```python
from build123d import *

# Parameters (mm, degrees)
SKETCH1_R                                    = 17.5
SKETCH1_R_2                                  = 8
BOSS_EXTRUDE1_DEPTH                          = 2
CSK_FOR_M3_COUNTERSUNK_FLAT_HEAD_SCR_2_COUNT = 2
CSK_FOR_M3_COUNTERSUNK_FLAT_HEAD_SCR_2_PITCH = 19.902355243
CSK_FOR_M3_COUNTERSUNK_FLAT_HEAD_SCR_3_COUNT = 2
CSK_FOR_M3_COUNTERSUNK_FLAT_HEAD_SCR_3_PITCH = 28.146180708
CSK_FOR_M3_COUNTERSUNK_FLAT_HEAD_SCR_4_COUNT = 2
CSK_FOR_M3_COUNTERSUNK_FLAT_HEAD_SCR_4_PITCH = 19.902355243


with BuildPart() as part:
    # Sketch1 → Boss-Extrude1 (new body)
    with BuildSketch(Plane.XY):
        Circle(SKETCH1_R)
        Circle(SKETCH1_R_2, mode=Mode.SUBTRACT)
    extrude(amount=BOSS_EXTRUDE1_DEPTH)

    # Sketch3 → CSK for M3 Countersunk Flat Head Screw1 (revolve, cut)
    with BuildSketch(Plane(origin=(0.559155654, 14.061977708, 0), x_dir=(0, 1, 0), z_dir=(1, 0, 0))):
        Polygon((0, 0), (0, 2), (1.7, 2), (1.7, 1.45), (3.15, 0), align=None)
    csk_for_m3_countersunk_flat_head_screw1 = revolve(axis=Axis((0.559155654, 14.061977708, -6.35), (0, 0, 1)), mode=Mode.SUBTRACT)

    # CSK for M3 Countersunk Flat Head Scr 2: CSK for M3 Countersunk Flat Head Screw1 ×2
    with Locations(*[Vector(-0.7346433717813886, -0.6784534739373604, 0) * (i * CSK_FOR_M3_COUNTERSUNK_FLAT_HEAD_SCR_2_PITCH) for i in range(1, CSK_FOR_M3_COUNTERSUNK_FLAT_HEAD_SCR_2_COUNT)]):
        add(csk_for_m3_countersunk_flat_head_screw1, mode=Mode.SUBTRACT)

    # CSK for M3 Countersunk Flat Head Scr 3: CSK for M3 Countersunk Flat Head Screw1 ×2
    with Locations(*[Vector(-0.03973225779969332, -0.9992103620810479, 0) * (i * CSK_FOR_M3_COUNTERSUNK_FLAT_HEAD_SCR_3_PITCH) for i in range(1, CSK_FOR_M3_COUNTERSUNK_FLAT_HEAD_SCR_3_COUNT)]):
        add(csk_for_m3_countersunk_flat_head_screw1, mode=Mode.SUBTRACT)

    # CSK for M3 Countersunk Flat Head Scr 4: CSK for M3 Countersunk Flat Head Screw1 ×2
    with Locations(*[Vector(0.6784534739373631, -0.7346433717813861, 0) * (i * CSK_FOR_M3_COUNTERSUNK_FLAT_HEAD_SCR_4_PITCH) for i in range(1, CSK_FOR_M3_COUNTERSUNK_FLAT_HEAD_SCR_4_COUNT)]):
        add(csk_for_m3_countersunk_flat_head_screw1, mode=Mode.SUBTRACT)


solid = part.part
```
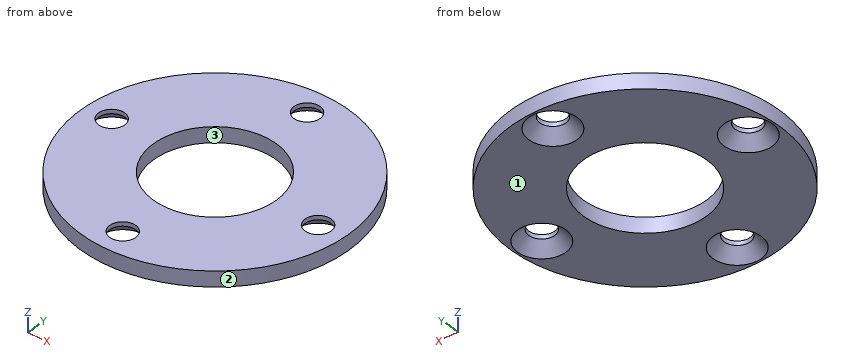
Work out the finished part from the listing and answer in its coordinate system (mm). Face numbers are marked on the shaded views. Give positions to 0.01 mm unless a question says otherwise; leave off trailing zeros. Write each loop counter-clockwise with the first axis right and the second up, starting at its lowest first coordinate (ties: lowest second). Pieces come first, ordered by that corner, then holes. Notation, with made-up numbers: (43, -10) -> (72, -10) arc R20 cw to (72, 0) -> close; hole circle Ø7 at (-25, 7). An arc over 180 degrees is marked (long way). Write each question's results on one line, items separated by ' | '.
1. Find section B-B on z = 0.35. Determine the outline of the cut face in (x, y), and give its area (3 significant figures).
Data:
outline: circle Ø35 at (0, 0); hole circle Ø5.6 at (-14.06, 0.56); hole circle Ø16 at (0, 0); hole circle Ø5.6 at (-0.56, -14.06); hole circle Ø5.6 at (0.56, 14.06); hole circle Ø5.6 at (14.06, -0.56) | area: 663 mm^2
2. Determine the mould class of the marked faces 1, 2 and 3 for opening direction Y: +Y half, -Y half, draft (parallel to the pull), parting line (faces both ways), or undercut.
Data:
face 1: draft | face 2: parting line | face 3: undercut
3. Find section D-D on x = 0. Give the number of separate pieces and of enclosed holes in the cut face, and give its area (3 significant figures).
Data:
separate pieces: 4 | enclosed holes: 0 | area: 20.8 mm^2
4. Find section A-A on x = -5. Determine the outline of the cut face in (y, z) (1 decimal).
Data:
outline: (-16.8, 0) -> (-6.2, 0) -> (-6.2, 2) -> (-16.8, 2) -> close; (6.2, 0) -> (16.8, 0) -> (16.8, 2) -> (6.2, 2) -> close
5. Straight lines are drawn through the part: L1, parallel to Y at x = -2, z = 1.8; L2, parallel to Y at x = 0, z = 0.95; L3, parallel to Y at x = 0, z = 0.65. For each, find the intervals that lie inside material, in ascending order.
Data:
L1: -17.39 to -14.96, -13.16 to -7.75, 7.75 to 17.39 | L2: -17.5 to -16.19, -11.93 to -8, 8 to 11.93, 16.19 to 17.5 | L3: -17.5 to -16.5, -11.63 to -8, 8 to 11.63, 16.5 to 17.5
6. This flat-tipped pin is pushed along its axis until it touches: pin 1 Ø5.5 at (x, y) = (0.56, 14.06) entering from +Z. Where does it stop, or does it pass through?
Data:
pin 1: z = 2
